Verification items for the finished model (mm, model axes). Coordinates: 2 decimals unless noted, no trailing zeros. Write each loop counter-clockwise with the first axis right and the second up, starting at its lowest first coordinate (ties: lowest second). Pieces come first, ordered by that corner, then holes. Notation, with made-up numbers: (27.25, 51.25) - (83.25, 51.25) arc R4 ccw to (83.25, 58.25) - close; hole circle Ø3 at (16.5, 59). An arc over 180 degrees is marked (long way). Use CSV: the item, a comma, the result in double quotes. Start each with the question number.
```python
from build123d import *

# Parameters (mm, degrees)
EXTRUDE_1_DEPTH     = 250
CUT_EXTRUDE_2_DEPTH = 7.5


with BuildPart() as part:
    # 草图1 → 凸台-拉伸1 (new body)
    with BuildSketch(Plane.XY):
        with BuildLine():
            Line((-17.5, 0), (-12.8, 0))
            ThreePointArc((-12.8, 0), (-12.234314575, 0.234314575), (-12, 0.8))
            Line((-12, 0.8), (-12, 5.2))
            ThreePointArc((-12, 5.2), (-11.765685425, 5.765685425), (-11.2, 6))
            Line((-11.2, 6), (11.2, 6))
            ThreePointArc((11.2, 6), (11.765685425, 5.765685425), (12, 5.2))
            Line((12, 5.2), (12, 0.8))
            ThreePointArc((12, 0.8), (12.234314575, 0.234314575), (12.8, 0))
            Line((12.8, 0), (17.5, 0))
            Line((17.5, 0), (17.5, 1.5))
            Line((17.5, 1.5), (14.3, 1.5))
            ThreePointArc((14.3, 1.5), (13.734314575, 1.734314575), (13.5, 2.3))
            Line((13.5, 2.3), (13.5, 6.7))
            ThreePointArc((13.5, 6.7), (13.265685425, 7.265685425), (12.7, 7.5))
            Line((12.7, 7.5), (-12.7, 7.5))
            ThreePointArc((-12.7, 7.5), (-13.265685425, 7.265685425), (-13.5, 6.7))
            Line((-13.5, 6.7), (-13.5, 2.3))
            ThreePointArc((-13.5, 2.3), (-13.734314575, 1.734314575), (-14.3, 1.5))
            Line((-14.3, 1.5), (-17.5, 1.5))
            Line((-17.5, 1.5), (-17.5, 0))
        make_face()
    extrude(amount=EXTRUDE_1_DEPTH)

    # 草图2 → 切除-拉伸2 (cut)
    with BuildSketch(Plane(origin=(0, 0, 0), x_dir=(1, 0, 0), z_dir=(0, 1, 0))):
        with BuildLine():
            Line((3.1, 4.4), (3.1, -4.4))
            ThreePointArc((3.1, -4.4), (0, -7.5), (-3.1, -4.4))
            Line((-3.1, -4.4), (-3.1, 4.4))
            ThreePointArc((-3.1, 4.4), (0, 7.5), (3.1, 4.4))
        make_face()
        with BuildLine():
            Line((3.1, -15.6), (3.1, -24.4))
            ThreePointArc((3.1, -24.4), (0, -27.5), (-3.1, -24.4))
            Line((-3.1, -24.4), (-3.1, -15.6))
            ThreePointArc((-3.1, -15.6), (0, -12.5), (3.1, -15.6))
        make_face()
        with BuildLine():
            Line((3.1, -35.6), (3.1, -44.4))
            ThreePointArc((3.1, -44.4), (0, -47.5), (-3.1, -44.4))
            Line((-3.1, -44.4), (-3.1, -35.6))
            ThreePointArc((-3.1, -35.6), (0, -32.5), (3.1, -35.6))
        make_face()
        with BuildLine():
            Line((3.1, -55.6), (3.1, -64.4))
            ThreePointArc((3.1, -64.4), (0, -67.5), (-3.1, -64.4))
            Line((-3.1, -64.4), (-3.1, -55.6))
            ThreePointArc((-3.1, -55.6), (0, -52.5), (3.1, -55.6))
        make_face()
        with BuildLine():
            Line((3.1, -75.6), (3.1, -84.4))
            ThreePointArc((3.1, -84.4), (0, -87.5), (-3.1, -84.4))
            Line((-3.1, -84.4), (-3.1, -75.6))
            ThreePointArc((-3.1, -75.6), (0, -72.5), (3.1, -75.6))
        make_face()
        with BuildLine():
            Line((3.1, -95.6), (3.1, -104.4))
            ThreePointArc((3.1, -104.4), (0, -107.5), (-3.1, -104.4))
            Line((-3.1, -104.4), (-3.1, -95.6))
            ThreePointArc((-3.1, -95.6), (0, -92.5), (3.1, -95.6))
        make_face()
        with BuildLine():
            Line((3.1, -115.6), (3.1, -124.4))
            ThreePointArc((3.1, -124.4), (0, -127.5), (-3.1, -124.4))
            Line((-3.1, -124.4), (-3.1, -115.6))
            ThreePointArc((-3.1, -115.6), (0, -112.5), (3.1, -115.6))
        make_face()
        with BuildLine():
            Line((3.1, -135.6), (3.1, -144.4))
            ThreePointArc((3.1, -144.4), (0, -147.5), (-3.1, -144.4))
            Line((-3.1, -144.4), (-3.1, -135.6))
            ThreePointArc((-3.1, -135.6), (0, -132.5), (3.1, -135.6))
        make_face()
        with BuildLine():
            Line((3.1, -155.6), (3.1, -164.4))
            ThreePointArc((3.1, -164.4), (0, -167.5), (-3.1, -164.4))
            Line((-3.1, -164.4), (-3.1, -155.6))
            ThreePointArc((-3.1, -155.6), (0, -152.5), (3.1, -155.6))
        make_face()
        with BuildLine():
            Line((3.1, -175.6), (3.1, -184.4))
            ThreePointArc((3.1, -184.4), (0, -187.5), (-3.1, -184.4))
            Line((-3.1, -184.4), (-3.1, -175.6))
            ThreePointArc((-3.1, -175.6), (0, -172.5), (3.1, -175.6))
        make_face()
        with BuildLine():
            Line((3.1, -195.6), (3.1, -204.4))
            ThreePointArc((3.1, -204.4), (0, -207.5), (-3.1, -204.4))
            Line((-3.1, -204.4), (-3.1, -195.6))
            ThreePointArc((-3.1, -195.6), (0, -192.5), (3.1, -195.6))
        make_face()
        with BuildLine():
            Line((3.1, -215.6), (3.1, -224.4))
            ThreePointArc((3.1, -224.4), (0, -227.5), (-3.1, -224.4))
            Line((-3.1, -224.4), (-3.1, -215.6))
            ThreePointArc((-3.1, -215.6), (0, -212.5), (3.1, -215.6))
        make_face()
        with BuildLine():
            Line((3.1, -235.6), (3.1, -244.4))
            ThreePointArc((3.1, -244.4), (0, -247.5), (-3.1, -244.4))
            Line((-3.1, -244.4), (-3.1, -235.6))
            ThreePointArc((-3.1, -235.6), (0, -232.5), (3.1, -235.6))
        make_face()
    extrude(amount=CUT_EXTRUDE_2_DEPTH, mode=Mode.SUBTRACT)


solid = part.part
```
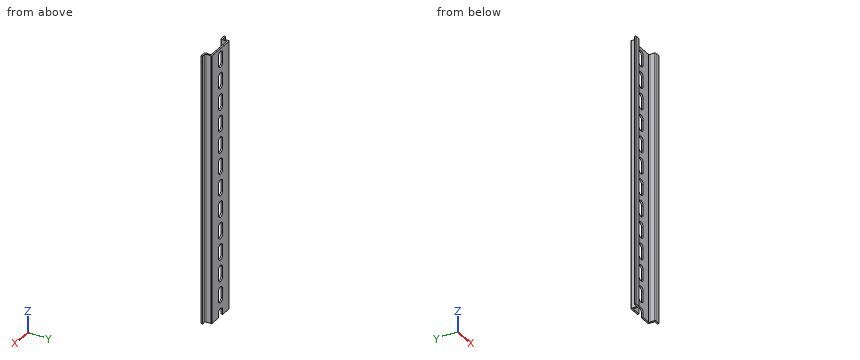
Q1. Gauge pin test, flat ends, axial feed: pin 1 (0.8 mm diameter, centred on y = 7, z = 140.5, fed in from -X); pin 2 (0.8 mm diameter, centred on y = 6.5, z = 21, fed in from +X); pin 3 (3.5 mm diameter, centred on y = 3.5, z = 176, fed in from +X); pin 4 (1.5 mm diameter, centred on x = 8.5, y = 4.5, fed in from +Z). Record the tip position at first contact, or that the pin passes through.
Q2. Cross-section at A-A (z = 101). Record the cut outline in (x, y), plus the area to 3 significant figures.
Q3. Scan lines: line 1 along X through (y, z) = (5.25, 54); line 2 along Y through (x, z) = (-5, 222.5); line 3 along X through (y, z) = (7, 139). Record each from-to range of solid material in increasing order. Write a range as from..to.
Q4. Cross-section at B-B (x = -8.5). Record the cut outline in (y, z), plus the area to 3 significant figures.
Reply:
1,pin 1,"x = -13.5"
1,pin 2,"x = 13.5"
1,pin 3,"x = 13.72"
1,pin 4,"through"
2,outline,"(-17.5, 0) - (-12.8, 0) arc R0.8 ccw to (-12, 0.8) - (-12, 5.2) arc R0.8 cw to (-11.2, 6) - (-3.1, 6) - (-3.1, 7.5) - (-12.7, 7.5) arc R0.8 ccw to (-13.5, 6.7) - (-13.5, 2.3) arc R0.8 cw to (-14.3, 1.5) - (-17.5, 1.5) - close; (3.1, 6) - (11.2, 6) arc R0.8 cw to (12, 5.2) - (12, 0.8) arc R0.8 ccw to (12.8, 0) - (17.5, 0) - (17.5, 1.5) - (14.3, 1.5) arc R0.8 cw to (13.5, 2.3) - (13.5, 6.7) arc R0.8 ccw to (12.7, 7.5) - (3.1, 7.5) - close"
2,area,"61.2 mm^2"
3,line 1,"-13.5..-12, 12..13.5"
3,line 2,"6..7.5"
3,line 3,"-13.44..-3.1, 3.1..13.44"
4,outline,"(6, 0) - (7.5, 0) - (7.5, 250) - (6, 250) - close"
4,area,"375 mm^2"
